Answer from the drawing. Dimensions are ordinates in mm from the lowest x, y and z of the part. Round coordinates to 2 decimals unless told otherwise and drop trailing zeros. Loops run counter-clockwise (first coordinate to the right, second up) from the corner with the lowest first, then second, coordinate; pieces in that order, holes last. Notation, with made-up numbers: (71, 15.5) - (86, 15.5) arc R20 ccw to (86, 53.5) - close; hole circle Ø4 at (71.25, -17). An arc over 180 degrees is marked (long way). Write item = value, one per line. Start each with the question number.
1) Section A-A, the plane y = 281 is taken. Determine the outline of the cut face in (x, z), and give its area (3 significant figures).
2) Straight lines are drawn through the part: line 1 along X through (y, z) = (629.5, 50.5); line 2 along Z through (x, y) = (53.5, 687). For each, find the intervals that lie inside material, in ascending order.
3) Section C-C, the plane x = 56.5 is taken. Determine the outline of the cut face in (y, z), and give its area (3 significant figures).
4) Given pin 1 Ø8 at (y, z) = (873.5, 8) entering from +X; pin 2 Ø8 at (x, y) = (35.5, 292.5) entering from -Z, each flat-ended and moving along its own axis, determine where each tip first touches the part or whether it passes through.
5) Section B-B, the plane z = 18 is taken. Determine the outline of the cut face in (x, y).
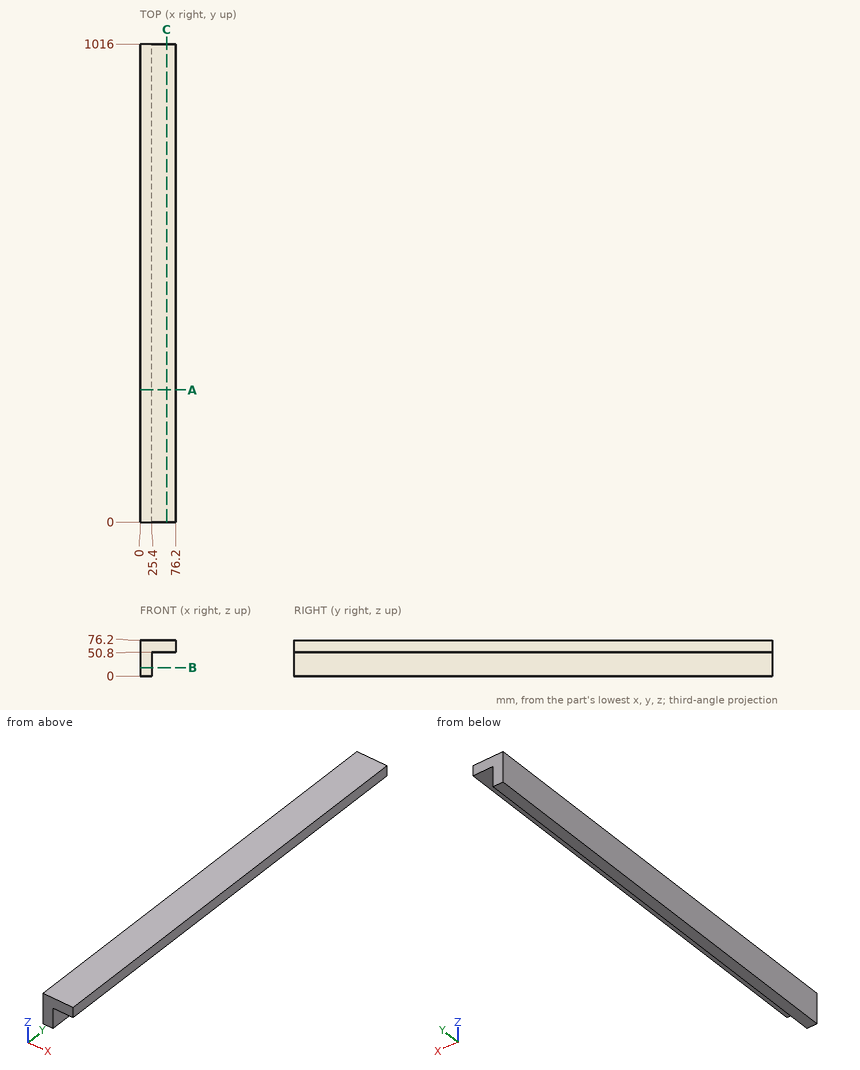
Geometry check:
q1.outline = (0, 0) - (25.4, 0) - (25.4, 50.8) - (76.2, 50.8) - (76.2, 76.2) - (0, 76.2) - close
q1.area = 3,230 mm2
q2.line_1 = 0 to 25.4
q2.line_2 = 50.8 to 76.2
q3.outline = (0, 50.8) - (1016, 50.8) - (1016, 76.2) - (0, 76.2) - close
q3.area = 25,800 mm2
q4.pin_1 = 25.4
q4.pin_2 = 50.8
q5.outline = (0, 0) - (25.4, 0) - (25.4, 1016) - (0, 1016) - close
